```python
from build123d import *

# Parameters (mm, degrees)
PAD_DEPTH       = 1.7
SKETCH003_W     = 5.61
SKETCH003_H     = 19.7
PAD008_DEPTH    = 13
SKETCH020_W     = 4.61
SKETCH020_H     = 11.65
SKETCH020_W_2   = 1
SKETCH020_H_2   = 10.75
POCKET009_DEPTH = 18
FILLET012_R     = 0.5
FILLET013_R     = 0.5
CHAMFER_SIZE    = 0.3


with BuildPart() as part:
    # Sketch → Pad (new body)
    with BuildSketch(Plane.XY):
        with BuildLine():
            Line((0, 0), (30, 0))
            Line((30, 0), (30, 1))
            Line((30, 1), (31, 1))
            Line((31, 1), (31, 18.27))
            Line((31, 18.27), (24.4, 18.27))
            ThreePointArc((24.4, 24.87), (21.1, 21.57), (24.4, 18.27))
            Line((24.4, 24.87), (31, 24.87))
            Line((31, 24.87), (31, 59.13))
            Line((31, 59.13), (24.4, 59.13))
            ThreePointArc((24.4, 65.73), (21.1, 62.43), (24.4, 59.13))
            Line((24.4, 65.73), (31, 65.73))
            Line((31, 65.73), (31, 83))
            Line((30, 83), (31, 83))
            Line((30, 84), (30, 83))
            Line((30, 84), (0, 84))
            Line((0, 84), (-30, 84))
            Line((-30, 84), (-30, 83))
            Line((-30, 83), (-31, 83))
            Line((-31, 83), (-31, 65.73))
            Line((-31, 65.73), (-24.4, 65.73))
            ThreePointArc((-24.4, 59.13), (-21.1, 62.43), (-24.4, 65.73))
            Line((-24.4, 59.13), (-31, 59.13))
            Line((-31, 59.13), (-31, 24.87))
            Line((-31, 24.87), (-24.4, 24.87))
            ThreePointArc((-24.4, 18.27), (-21.1, 21.57), (-24.4, 24.87))
            Line((-24.4, 18.27), (-31, 18.27))
            Line((-31, 18.27), (-31, 1))
            Line((-31, 1), (-30, 1))
            Line((-30, 1), (-30, 0))
            Line((-30, 0), (0, 0))
        make_face()
    extrude(amount=PAD_DEPTH)

    # Sketch003 → Pad008 (new body)
    with BuildSketch(Plane.XY.offset(1.7)):
        with Locations((-4.675, 78.17)):
            Rectangle(SKETCH003_W, SKETCH003_H)
        with Locations((4.975, 78.17)):
            Rectangle(SKETCH003_W, SKETCH003_H)
    extrude(amount=PAD008_DEPTH)

    # Sketch020 → Pocket009 (cut)
    with BuildSketch(Plane(origin=(0, 88.02, 0), x_dir=(-1, 0, 0), z_dir=(0, 1, 0))):
        with Locations((-4.975, 8.375)):
            Rectangle(SKETCH020_W, SKETCH020_H)
        with Locations((-6.28, 8.325)):
            Rectangle(SKETCH020_W_2, SKETCH020_H_2, mode=Mode.SUBTRACT)
        with Locations((4.675, 8.375)):
            Rectangle(SKETCH020_W, SKETCH020_H)
        with Locations((3.37, 8.325)):
            Rectangle(SKETCH020_W_2, SKETCH020_H_2, mode=Mode.SUBTRACT)
    extrude(amount=-POCKET009_DEPTH, mode=Mode.SUBTRACT)

    # Fillet012
    fillet012_edges = [part.edges().sort_by_distance(p)[0] for p in [
        (7.78, 78.17, 14.7),
        (2.17, 78.17, 14.7),
        (-1.87, 78.17, 14.7),
        (-7.48, 78.17, 14.7),
        (-7.48, 86.01, 1.7),
        (2.17, 86.01, 1.7),
        (7.78, 86.01, 1.7),
        (-1.87, 86.01, 1.7),
    ]]
    fillet(fillet012_edges, radius=FILLET012_R)

    # Fillet013
    fillet013_edges = [part.edges().sort_by_distance(p)[0] for p in [
        (7.28, 79.02, 14.2),
        (-2.37, 79.02, 14.2),
        (2.67, 79.02, 14.2),
        (-6.98, 79.02, 14.2),
        (7.28, 79.02, 2.55),
        (-2.37, 79.02, 2.55),
        (2.67, 79.02, 2.55),
        (-6.98, 79.02, 2.55),
    ]]
    fillet(fillet013_edges, radius=FILLET013_R)

    # Chamfer
    chamfer_edges = [part.edges().sort_by_distance(p)[0] for p in [
        (6.78, 79.02, 13.7),
        (-2.87, 79.02, 13.7),
        (-2.87, 79.02, 2.95),
        (6.78, 79.02, 2.95),
    ]]
    chamfer(chamfer_edges, length=CHAMFER_SIZE)


solid = part.part
```
Input: part model. Units: mm. Frame: model coordinates. A direction names the side the tool comes from. Round coordinates to 2 decimals unless told otherwise and drop trailing zeros. Loops run counter-clockwise (first coordinate to the right, second up) from the corner with the lowest first, then second, coordinate; pieces in that order, holes last. Notation, with made-up numbers: (-10, -21.5) - (-2, -21.5) arc R31 ccw to (-2, 5.5) - close; hole circle Ø10 at (79.25, 55.5). An arc over 180 degrees is marked (long way). One line per item, written item: value. Start each with the question number.
(1) Access query for faces 1 (the flat face through (-7.48, 78, 8)), 2 (the flat face through (7.78, 78, 8)), 3 (the flat face through (-28, 18.27, 1)), 4 (the flat face through (28, 18.27, 1)), 5 (the flat face through (-2.87, 79, 8)). Directions: +Z, -Z, +X, -X, +Y, -Y. A direction counts if a zero-diameter tool reaches every point of the face in a straight line with its end or side. Return the directions, or none.
(2) Section C-C, the plane x = -19. Return loops of the section in (y, z).
(3) Ray query, line 1 (X direction, y = 68.5, z = 7.5); line 2 (Z direction, x = -6.5, y = 46); line 3 (Y direction, x = 13, z = 1). Return the intervals inside material, ascending. Write a range as [from, to].
(4) Draft query along Z for faces 6 (the flat face through (5, 86, 1.7)), 7 (the flat face through (0, 84, 1)), 8 (the flat face through (7.28, 79, 8)), 9 (the flat face through (4, 70.02, 8)). Return one class per face: +Z half, -Z half, draft (parallel to the pull), parting line (faces both ways), or undercut.
(5) Section B-B, the plane y = 81.5. Count the separate pieces of the cut face and the enclosed holes in it, plus the area to 3 significant figures.
(6) Section A-A, the plane z = 7.75. Return loops of the section in (x, y), plus the area to 3 significant figures.
(7) Contact query for flat-ended pins moving along their axis: P1, Ø1.4, axis at x = 26, z = 1, coming from the +Y side; P2, Ø10, axis at x = -12, y = 12, coming from the +Z side; P3, Ø4, axis at y = 82, z = 9.5, coming from the -X side; P4, Ø12, axis at x = 21.5, y = 12, coming from the -Z side. Output: stop coordinate, or through.
(8) Section D-D, the plane y = 21.57. Return loops of the section in (x, z).
Results below:
1. face 1: +Z, -X, +Y, -Y
1. face 2: +Z, +X, +Y, -Y
1. face 3: +Z, -Z, -X
1. face 4: +Z, -Z, +X
1. face 5: +Y
2. outline: (0, 0) - (84, 0) - (84, 1.7) - (0, 1.7) - close
3. line 1: [-7.48, -1.87], [2.17, 7.78]
3. line 2: [0, 1.7]
3. line 3: [0, 84]
4. face 6: -Z half
4. face 7: draft
4. face 8: undercut
4. face 9: undercut
5. separate pieces: 3
5. enclosed holes: 2
5. area: 165 mm^2
6. outline: (-7.48, 68.32) - (-1.87, 68.32) - (-1.87, 88.02) - (-2.37, 88.02) - (-2.37, 70.02) - (-2.87, 70.02) - (-2.87, 88.02) - (-3.87, 88.02) - (-3.87, 70.02) - (-6.98, 70.02) - (-6.98, 88.02) - (-7.48, 88.02) - close; (2.17, 68.32) - (7.78, 68.32) - (7.78, 88.02) - (7.28, 88.02) - (7.28, 70.02) - (6.78, 70.02) - (6.78, 88.02) - (5.78, 88.02) - (5.78, 70.02) - (2.67, 70.02) - (2.67, 88.02) - (2.17, 88.02) - close
6. area: 91.1 mm^2
7. P1: y = 84
7. P2: z = 1.7
7. P3: x = -7.48
7. P4: z = 0
8. outline: (-21.1, 0) - (21.1, 0) - (21.1, 1.7) - (-21.1, 1.7) - close
